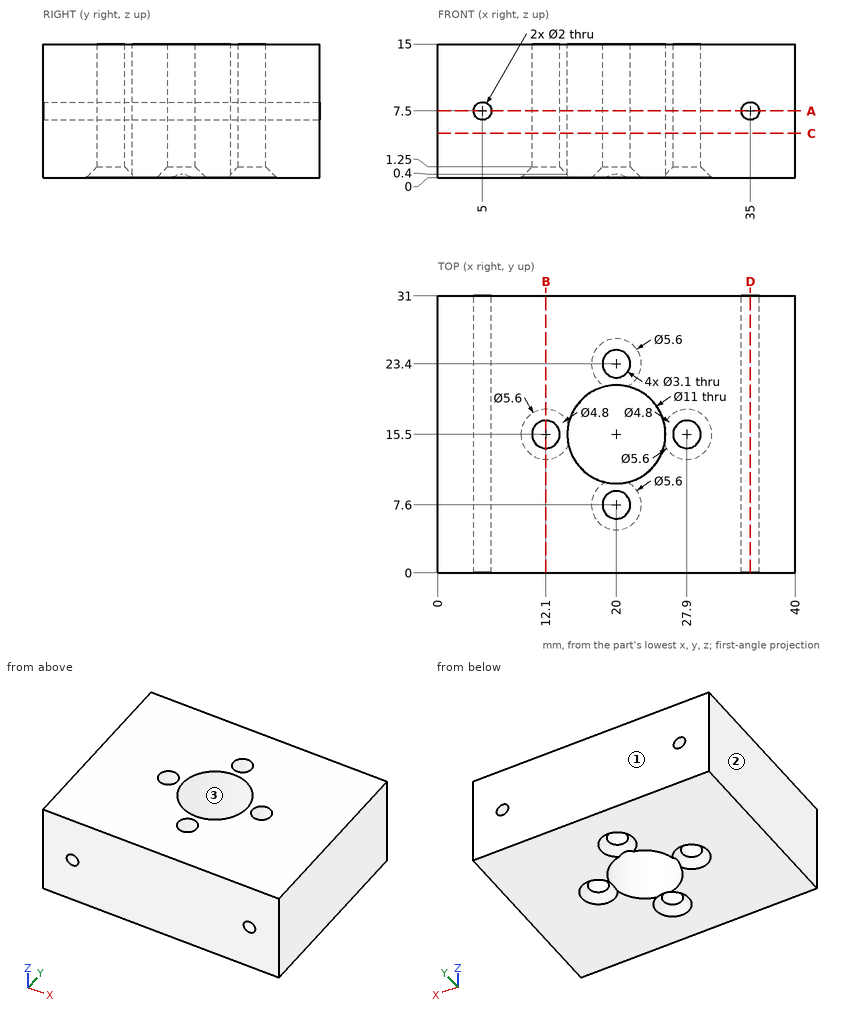
Can you work these out from the drawing? Everything is in mm from the part's minimum corner. Coordinates: 2 decimals unless noted, no trailing zeros. Loops run counter-clockwise (first coordinate to the right, second up) from the corner with the lowest first, then second, coordinate; pieces in that order, holes last.
1) Imagine slicing it at A-A on z = 7.5. List the corners of the cut face in (x, y) for me, plus the area to 3 significant figures.
2) Thinking about a two-plate mould opening in X: for the marked faces 1, 2 and 3, which applies, pulls with the +X half, pulls with the -X half, needs draft (parallel to the pull), parting line crosses it, or undercut?
3) For pin 1 (4 mm diameter, centred on x = 20, y = 7.6, fed in from -Z), with a flat end and sliding along its axis, tell me the tip position at first contact or that it passes through.
4) I need wall thicknesses on probe 1 along Y at (x, z) = (20, 8); probe 2 along Z at (x, y) = (5, 18); probe 3 along Y at (x, z) = (12.1, 12). Which ranges of each line are inside material? Lowest first, please.
5) Imagine slicing it at D-D on x = 35. List the corners of the cut face in (y, z) for me, plus the area to 3 significant figures.
6) Imagine slicing it at C-C on z = 5. List the corners of the cut face in (x, y) for me, plus the area to 3 significant figures.
7) Imagine slicing it at B-B on x = 12.1. List the corners of the cut face in (y, z) for me.
Completed:
1. outline: (0, 0) - (4, 0) - (4, 31) - (0, 31) - close; (6, 0) - (34, 0) - (34, 31) - (6, 31) - close; (36, 0) - (40, 0) - (40, 31) - (36, 31) - close; hole circle Ø3.1 at (12.1, 15.5); hole circle Ø11 at (20, 15.5); hole circle Ø3.1 at (20, 7.6); hole circle Ø3.1 at (20, 23.4); hole circle Ø3.1 at (27.9, 15.5)
1. area: 991 mm2
2. face 1: needs draft
2. face 2: pulls with the -X half
2. face 3: undercut
3. pin 1: stops at z = 0.8
4. probe 1: y = 0 to 6.05, 9.15 to 10, 21 to 21.85, 24.95 to 31
4. probe 2: z = 0 to 6.5, 8.5 to 15
4. probe 3: y = 0 to 13.95, 17.05 to 31
5. outline: (0, 0) - (31, 0) - (31, 6.5) - (0, 6.5) - close; (0, 8.5) - (31, 8.5) - (31, 15) - (0, 15) - close
5. area: 403 mm2
6. outline: (0, 0) - (40, 0) - (40, 31) - (0, 31) - close; hole circle Ø3.1 at (12.1, 15.5); hole circle Ø11 at (20, 15.5); hole circle Ø3.1 at (20, 7.6); hole circle Ø3.1 at (20, 23.4); hole circle Ø3.1 at (27.9, 15.5)
6. area: 1,110 mm2
7. outline: (0, 0) - (12.7, 0) - (13.95, 1.25) - (13.95, 15) - (0, 15) - close; (17.05, 1.25) - (18.3, 0) - (31, 0) - (31, 15) - (17.05, 15) - close
